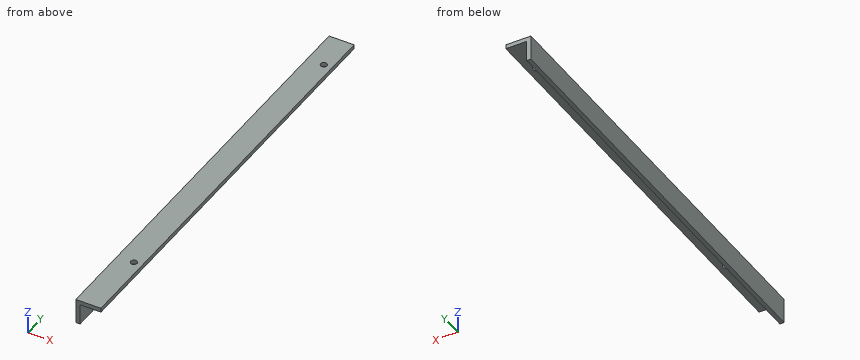
from build123d import *

# Parameters (mm, degrees)
BOSS_EXTRUDE1_DEPTH = 330.2
CUT_EXTRUDE1_REACH  = 333.13
SKETCH2_R           = 2.413


with BuildPart() as part:
    # Sketch1 → Boss-Extrude1 (new body)
    with BuildSketch(Plane(origin=(0, 0, 0), x_dir=(1, 0, 0), z_dir=(0, 1, 0))):
        Polygon((3.175, 3.175), (3.175, 19.05), (0, 19.05), (0, 0), (19.05, 0), (19.05, 3.175), align=None)
    extrude(amount=BOSS_EXTRUDE1_DEPTH)

    # Sketch2 → Cut-Extrude1 (cut, up to next)
    with BuildSketch(Plane(origin=(0, 0, -3.175), x_dir=(-1, 0, 0), z_dir=(0, 0, -1)), mode=Mode.PRIVATE) as cut_extrude1_sk1:
        with Locations((-12.7, 53.975)):
            Circle(SKETCH2_R)
    cut_extrude1_tool1 = extrude(cut_extrude1_sk1.sketch, amount=-CUT_EXTRUDE1_REACH, mode=Mode.PRIVATE) & part.part
    # Sketch2 → Cut-Extrude1 (cut, up to next)
    with BuildSketch(Plane(origin=(0, 0, -3.175), x_dir=(-1, 0, 0), z_dir=(0, 0, -1)), mode=Mode.PRIVATE) as cut_extrude1_sk2:
        with Locations((-12.7, 301.625)):
            Circle(SKETCH2_R)
    cut_extrude1_tool2 = extrude(cut_extrude1_sk2.sketch, amount=-CUT_EXTRUDE1_REACH, mode=Mode.PRIVATE) & part.part
    add(cut_extrude1_tool1.solids().sort_by_distance((12.7, 53.975, -3.175))[0], mode=Mode.SUBTRACT)
    add(cut_extrude1_tool2.solids().sort_by_distance((12.7, 301.625, -3.175))[0], mode=Mode.SUBTRACT)


solid = part.part
Geometry check sheet. Reference: the model listing, model coordinates, mm. Coordinates: 2 decimals unless noted, no trailing zeros. Order: outer loops, then holes, each group sorted by start corner. A loop starts at its lowest first (then second) coordinate and runs counter-clockwise, first axis right, second up. Notation, with made-up numbers: (-23, 58) - (34, 58) arc R6 ccw to (34, 68) - close; hole circle Ø2 at (25.25, 52). An arc over 180 degrees is marked (long way). Answer in a Markdown table with one row per item. Add a question column.
1) Cross-section at A-A, the plane y = 46.5. Record the cut outline in (x, z) (3 decimals), then the cut area to 3 significant figures.
2) Material ranges on line 1 along Y through (x, z) = (12.7, -2.4); line 2 along Z through (x, y) = (5.25, 123) (3 decimals); line 3 along X through (y, z) = (274, -13.5) (3 decimals), recorded low to high. Write a range as [from, to].
3) Cross-section at B-B, the plane z = -12.75. Record the cut outline in (x, y) (3 decimals).
4) Gauge pin test, flat ends, axial feed: P1, Ø1.5, axis at x = 12, y = 135, coming from the -Z side (3 decimals); P2, Ø5, axis at y = 126, z = -8, coming from the +X side (3 decimals). Record the tip position at first contact, or that the pin passes through.
5) Cross-section at C-C, the plane x = 7.25. Record the cut outline in (y, z) (3 decimals), then the cut area to 3 significant figures.
Check result:
| question | item | result |
|---|---|---|
| 1 | outline | (0, -19.05) - (3.175, -19.05) - (3.175, -3.175) - (19.05, -3.175) - (19.05, 0) - (0, 0) - close |
| 1 | area | 111 mm² |
| 2 | line 1 | y = [0, 51.56], [56.39, 299.21], [304.04, 330.2] |
| 2 | line 2 | z = [-3.175, 0] |
| 2 | line 3 | x = [0, 3.175] |
| 3 | outline | (0, 0) - (3.175, 0) - (3.175, 330.2) - (0, 330.2) - close |
| 4 | P1 | stops at z = -3.175 |
| 4 | P2 | stops at x = 3.175 |
| 5 | outline | (0, -3.175) - (330.2, -3.175) - (330.2, 0) - (0, 0) - close |
| 5 | area | 1,050 mm² |
